Read the model definition and answer for the solid it produces. Units are mm, in the model's axes. Give positions to 0.01 mm unless a question says otherwise; leave off trailing zeros. Loops run counter-clockwise (first coordinate to the right, second up) from the corner with the lowest first, then second, coordinate; pieces in that order, holes last. Notation, with made-up numbers: (-3.5, -10) - (42.5, -10) arc R19 ccw to (42.5, 17) - close; hole circle Ø2 at (49, -40). An arc over 180 degrees is marked (long way). Use a Markdown table: item, result. Add a question column.
Item 1: A cutting plane is placed at B-B (z = -7.25). Determine the outline of the cut face in (x, y), plus the area to 3 significant figures.
Item 2: A cutting plane is placed at A-A (y = 0). Give the number of separate pieces and of enclosed holes in the cut face, plus the area to 3 significant figures.
Item 3: A cutting plane is placed at C-C (x = 107.5). Determine the outline of the cut face in (y, z).
Item 4: Each of these flat-tipped pins is pushed along its axis until it touches: P1, Ø3.5, axis at y = 2, z = -8.5, coming from the +X side; P2, Ø1.5, axis at y = 15, z = -10.5, coming from the -X side; P3, Ø1.5, axis at y = -18.5, z = -6, coming from the -X side. Where does it stop, or does it pass through?
Item 5: Consider probe 1 along Y at (x, z) = (204.48, -7.5); probe 2 along Y at (x, z) = (56, -3.75); probe 3 along Y at (x, z) = (53, -2.75). Determine where each line is inside the solid, lowest interval first. Write a range as [from, to].
from build123d import *

# Parameters (mm, degrees)
BOSS_EXTRUDE2_DEPTH = 12
CUT_EXTRUDE4_DEPTH  = 12
SKETCH8_R           = 20.1
CUT_EXTRUDE5_DEPTH  = 19
SKETCH9_R           = 20.1
CUT_EXTRUDE6_DEPTH  = 19


with BuildPart() as part:
    # Sketch1 → Boss-Extrude2 (new body)
    with BuildSketch(Plane.XY):
        with BuildLine():
            Line((0, 29.5), (204.48, 29.5))
            ThreePointArc((204.48, 29.5), (233.98, 0), (204.48, -29.5))
            Line((204.48, -29.5), (0, -29.5))
            ThreePointArc((0, -29.5), (-29.5, 0), (0, 29.5))
        make_face()
    extrude(amount=-BOSS_EXTRUDE2_DEPTH)

    # Sketch7 → Cut-Extrude4 (cut)
    with BuildSketch(Plane.XY):
        with BuildLine():
            Line((56.938938215, -17.5), (36.938938215, 17.5))
            ThreePointArc((36.938938215, 17.5), (31.282083966, 15.156854249), (28.938938215, 9.5))
            Line((28.938938215, 9.5), (28.938938215, -9.5))
            ThreePointArc((28.938938215, -9.5), (31.282083966, -15.156854249), (36.938938215, -17.5))
            Line((36.938938215, -17.5), (56.938938215, -17.5))
        make_face()
        Polygon((88.938938215, 17.5), (48.938938215, 17.5), (68.938938215, -17.5), align=None)
        Polygon((120.938938215, -17.5), (100.938938215, 17.5), (80.938938215, -17.5), align=None)
        Polygon((152.938938215, 17.5), (112.938938215, 17.5), (132.938938215, -17.5), align=None)
        with BuildLine():
            Line((167.541061785, 17.5), (164.938938215, 17.5))
            Line((164.938938215, 17.5), (144.938938215, -17.5))
            Line((144.938938215, -17.5), (167.541061785, -17.5))
            ThreePointArc((167.541061785, -17.5), (173.197916034, -15.156854249), (175.541061785, -9.5))
            Line((175.541061785, -9.5), (175.541061785, 9.5))
            ThreePointArc((175.541061785, 9.5), (173.197916034, 15.156854249), (167.541061785, 17.5))
        make_face()
    extrude(amount=-CUT_EXTRUDE4_DEPTH, mode=Mode.SUBTRACT)

    # Sketch8 → Cut-Extrude5 (cut)
    with BuildSketch(Plane.XY):
        Circle(SKETCH8_R)
    extrude(amount=-CUT_EXTRUDE5_DEPTH, mode=Mode.SUBTRACT)

    # Sketch9 → Cut-Extrude6 (cut)
    with BuildSketch(Plane.XY):
        with Locations((204.48, 0)):
            Circle(SKETCH9_R)
    extrude(amount=-CUT_EXTRUDE6_DEPTH, mode=Mode.SUBTRACT)


solid = part.part
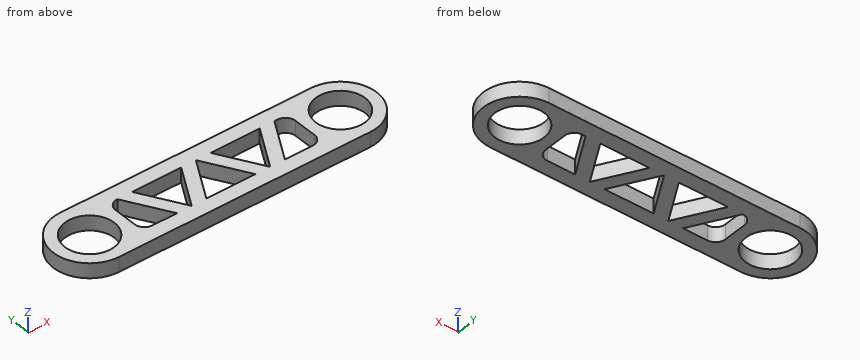
Geometry says:
| question | item | result |
|---|---|---|
| 1 | outline | (0, -29.5) - (204.48, -29.5) arc R29.5 ccw to (204.48, 29.5) - (0, 29.5) arc R29.5 ccw to start; hole circle Ø40.2 at (0, 0); hole (28.94, -9.5) arc R8 ccw to (36.94, -17.5) - (56.94, -17.5) - (36.94, 17.5) arc R8 ccw to (28.94, 9.5) - close; hole (48.94, 17.5) - (68.94, -17.5) - (88.94, 17.5) - close; hole (80.94, -17.5) - (120.94, -17.5) - (100.94, 17.5) - close; hole (112.94, 17.5) - (132.94, -17.5) - (152.94, 17.5) - close; hole (144.94, -17.5) - (167.54, -17.5) arc R8 ccw to (175.54, -9.5) - (175.54, 9.5) arc R8 ccw to (167.54, 17.5) - (164.94, 17.5) - close; hole circle Ø40.2 at (204.48, 0) |
| 1 | area | 8,860 mm² |
| 2 | separate pieces | 8 |
| 2 | enclosed holes | 0 |
| 2 | area | 1,010 mm² |
| 3 | outline | (-29.5, -12) - (-17.5, -12) - (-17.5, 0) - (-29.5, 0) - close; (6.02, -12) - (29.5, -12) - (29.5, 0) - (6.02, 0) - close |
| 4 | P1 | x = 233.98 |
| 4 | P2 | x = -25.83 |
| 4 | P3 | x = -23.56 |
| 5 | probe 1 | [-29.5, -20.1], [20.1, 29.5] |
| 5 | probe 2 | [-29.5, -17.5], [-15.86, 5.14], [17.5, 29.5] |
| 5 | probe 3 | [-29.5, -17.5], [-10.61, 10.39], [17.5, 29.5] |
